Geometry: final body of the model. Coordinates: model frame, mm. A direction names the side the tool comes from. Give positions to 0.01 mm unless a question says otherwise; leave off trailing zeros. Write each loop counter-clockwise with the first axis right and the second up, starting at its lowest first coordinate (ties: lowest second). Pieces come first, ordered by that corner, then holes. Notation, with made-up numbers: (84.5, -13.75) -> (134.5, -13.75) arc R18 ccw to (134.5, 1.25) -> close; hole circle Ø11 at (15, -7). An arc over 180 degrees is marked (long way). Answer as a JSON object with one key per item and string values.
from build123d import *

# Parameters (mm, degrees)
BOSS_EXTRUDE1_DEPTH = 5.68
SKETCH2_OUTSIDE_W   = 44.722
SKETCH2_OUTSIDE_H   = 42.972
SKETCH2_OUTSIDE_R   = 7.837529904
CUT_EXTRUDE1_DEPTH  = 5.68
CUT_EXTRUDE1_DRAFT  = -60
SKETCH3_R           = 4.5
BOSS_EXTRUDE2_DEPTH = 52


with BuildPart() as part:
    # Sketch1 → Boss-Extrude1 (new body)
    with BuildSketch(Plane.XY):
        Polygon((5.091015355, 7.482249839), (-3.934310761, 8.150073548), (-9.025326116, 0.667823708), (-5.091015355, -7.482249839), (3.934310761, -8.150073548), (9.025326116, -0.667823708), align=None)
    extrude(amount=BOSS_EXTRUDE1_DEPTH)


with BuildPart() as cut_extrude1_tool:
    # Sketch2 outside → Cut-Extrude1 (with draft: the straight prism first)
    with BuildSketch(Plane.XY.offset(5.68)):
        Rectangle(SKETCH2_OUTSIDE_W, SKETCH2_OUTSIDE_H)
        Circle(SKETCH2_OUTSIDE_R, mode=Mode.SUBTRACT)
    extrude(amount=-CUT_EXTRUDE1_DEPTH)
    # Cut-Extrude1: the draft: its side faces are tilted about the plane it starts from
    cut_extrude1_sides = [cut_extrude1_tool.faces().sort_by_distance(p)[0] for p in [
        (0, -21.486, 2.84),
        (22.361, 0, 2.84),
        (0, 21.486, 2.84),
        (-22.361, 0, 2.84),
        (-7.837529904, 0, 2.84),
    ]]
    draft(cut_extrude1_sides, Plane.XY.offset(5.68), CUT_EXTRUDE1_DRAFT)


with BuildPart() as part_1:
    add(part.part)

    # Cut-Extrude1: cut by cut_extrude1_tool
    add(cut_extrude1_tool.part, mode=Mode.SUBTRACT)

    # Sketch3 → Boss-Extrude2 (add)
    with BuildSketch(Plane(origin=(0, 0, 0), x_dir=(-1, 0, 0), z_dir=(0, 0, -1))):
        with Locations(Location((0, 0, 0), (0, 0, 180))):
            Circle(SKETCH3_R)
    extrude(amount=BOSS_EXTRUDE2_DEPTH)


solid = part_1.part
Q1. Set-up query: faces 1 (the cylindrical face through (-3.32, -3.04, -25.64)), 2 (the flat face through (-6.444, 4.461, 2.8)). Return all of +Z, -Z, +X, -X, +Y, -Y with unobstructed straight access to the full face (end or side cutting, diameter ignored); none if empty.
Values:
{"face 1": "-Z", "face 2": "+Z, -Z, -X, +Y"}
Q2. Cut plane B-B (y = 0). Return the cut outline in (x, z).
Values:
{"outline": "(-8.7, 0) -> (-4.5, 0) -> (-4.5, -52) -> (4.5, -52) -> (4.5, 0) -> (8.7, 0) -> (8.7, 5.18) -> (7.84, 5.68) -> (-7.84, 5.68) -> (-8.7, 5.18) -> close"}
Q3. Material intervals for L1, parallel to Z at x = 7.5, y = -0.25; L2, parallel to X at y = -3, z = -44; L3, parallel to Z at x = -8, y = 1.5, sorted ascending. Write a range as from..to.
Values:
{"L1": "0..5.68", "L2": "-3.35..3.35", "L3": "0..5.51"}
Q4. Cut plane C-C (z = -40.5). Return the cut outline in (x, y), and give its area (3 significant figures).
Values:
{"outline": "circle Ø9 at (0, 0)", "area": "63.6 mm²"}
Q5. First-contact query: P1, Ø3, axis at x = -1, z = -22, coming from the -Y side; P2, Ø8, axis at x = -6, z = -45.5, coming from the -Y side; P3, Ø3, axis at y = -5, z = -29, coming from the +X side. Flat tips, straight axial feed; report the tip coordinate or a pass-through.
Values:
{"P1": "y = -4.5", "P2": "y = -4.03", "P3": "x = 2.83"}
